CAD build for the part. Positions are in the model's coordinates, mm. A direction names the side the tool comes from. Give positions to 0.01 mm unless a question says otherwise; leave off trailing zeros. Loops run counter-clockwise (first coordinate to the right, second up) from the corner with the lowest first, then second, coordinate; pieces in that order, holes last. Notation, with made-up numbers: (5.5, 62.5) - (31.5, 62.5) arc R28 cw to (31.5, 86.5) - close; hole circle Ø11 at (5.5, 10). An arc over 180 degrees is marked (long way). Return JSON: item names as keys, results as strings.
from build123d import *

# Parameters (mm, degrees)
SKETCH3_R           = 30.358351357
BOSS_EXTRUDE2_DEPTH = 10
SKETCH4_R           = 26.969977479
SKETCH4_R_2         = 23.969977479
BOSS_EXTRUDE3_DEPTH = 30


with BuildPart() as part:
    # Sketch3 → Boss-Extrude2 (new body)
    with BuildSketch(Plane.XY):
        with Locations((-22.75, 10.5)):
            Circle(SKETCH3_R)
        with BuildLine():
            ThreePointArc((-35, 1.680276087), (-43.819723913, 10.5), (-35, 19.319723913))
            Line((-35, 19.319723913), (-28.378131485, 19.319723913))
            Line((-28.378131485, 19.319723913), (-28.378131485, 21))
            Line((-28.378131485, 21), (-17.074172485, 21))
            Line((-17.074172485, 21), (-17.074172485, 19.319723913))
            Line((-17.074172485, 19.319723913), (-10.5, 19.319723913))
            ThreePointArc((-10.5, 19.319723913), (-1.680276087, 10.5), (-10.5, 1.680276087))
            Line((-10.5, 1.680276087), (-16.75, 1.680276087))
            Line((-16.75, 1.680276087), (-16.75, 0))
            Line((-16.75, 0), (-28.75, 0))
            Line((-28.75, 0), (-28.75, 1.680276087))
            Line((-28.75, 1.680276087), (-35, 1.680276087))
        make_face(mode=Mode.SUBTRACT)
    extrude(amount=BOSS_EXTRUDE2_DEPTH)

    # Sketch4 → Boss-Extrude3 (add)
    with BuildSketch(Plane.XY.offset(10)):
        with Locations((-22.75, 10.5)):
            Circle(SKETCH4_R)
        with Locations((-22.75, 10.5)):
            Circle(SKETCH4_R_2, mode=Mode.SUBTRACT)
    extrude(amount=BOSS_EXTRUDE3_DEPTH)


solid = part.part
1. Cut at C-C, the plane z = 22. Write the cut outline in (x, y), plus the area to 3 significant figures.
Values follow:
{"outline": "circle Ø53.94 at (-22.75, 10.5); hole circle Ø47.94 at (-22.75, 10.5)", "area": "480 mm²"}
2. Cut at A-A, the plane x = -20. Write the cut outline in (y, z), plus the area to 3 significant figures.
Values follow:
{"outline": "(-19.73, 0) - (0, 0) - (0, 10) - (-13.31, 10) - (-13.31, 40) - (-16.33, 40) - (-16.33, 10) - (-19.73, 10) - close; (21, 0) - (40.73, 0) - (40.73, 10) - (37.33, 10) - (37.33, 40) - (34.31, 40) - (34.31, 10) - (21, 10) - close", "area": "576 mm²"}
3. Cut at D-D, the plane y = 28.5. Write the cut outline in (x, z), plus the area to 3 significant figures.
Values follow:
{"outline": "(-47.2, 0) - (1.7, 0) - (1.7, 10) - (-2.67, 10) - (-2.67, 40) - (-6.92, 40) - (-6.92, 10) - (-38.58, 10) - (-38.58, 40) - (-42.83, 40) - (-42.83, 10) - (-47.2, 10) - close", "area": "744 mm²"}
4. Drill centre lines: probe 1 along Y at (x, z) = (-22.75, 17.75); probe 2 along X at (y, z) = (10, 21); probe 3 along Z at (x, y) = (-26.5, 23.5). Where is each one in solid material? Low to high.
Values follow:
{"probe 1": "y = -16.47 to -13.47, 34.47 to 37.47", "probe 2": "x = -49.72 to -46.71, 1.21 to 4.22", "probe 3": "z = 0 to 10"}
5. Pull direction X, two halves, no side cores. Call faces 4 (the face through (-23, 38, 10)), 5 (the face through (-43.818, 10.306, 4.93)), 6 (the face through (-16.75, 1, 5)), 7 (the face through (2.975, 18.601, 24.79)): +X half, -X half, draft (parallel to the pull), parting line (faces both ways), or undercut.
Values follow:
{"face 4": "draft", "face 5": "undercut", "face 6": "undercut", "face 7": "parting line"}
6. Which spindle directions (+Z, -Z, +X, -X, +Y, -Y) get a long thin tool onto all of the face, cutting with end or side? Do faces 1 (the face through (-32, 1.68, 5)), 2 (the face through (-23, -3, 0)), 3 (the face through (0.113, 17.7, 24.79)). Say none if no direction does.
Values follow:
{"face 1": "+Z, -Z", "face 2": "-Z, +X, -X, +Y, -Y", "face 3": "+Z"}
7. Cut at B-B, the plane y = 10.5. Write the cut outline in (x, z), plus the area to 3 significant figures.
Values follow:
{"outline": "(-53.11, 0) - (-43.82, 0) - (-43.82, 10) - (-46.72, 10) - (-46.72, 40) - (-49.72, 40) - (-49.72, 10) - (-53.11, 10) - close; (-1.68, 0) - (7.61, 0) - (7.61, 10) - (4.22, 10) - (4.22, 40) - (1.22, 40) - (1.22, 10) - (-1.68, 10) - close", "area": "366 mm²"}
8. Drop flat-ended pins along their axis: P1, Ø11, axis at x = -24, z = 5.5, coming from the -Y side; P2, Ø3, axis at y = 32.5, z = 29, coming from the -X side; P3, Ø3, axis at y = 34, z = 27, coming from the +X side; P4, Ø14.5, axis at x = -23.5, y = 11, coming from the +Z side. Give the stop position or say it passes through.
Values follow:
{"P1": "stops at y = -19.86", "P2": "stops at x = -40.28", "P3": "stops at x = -7.15", "P4": "passes through"}
